The model under review builds one solid part; all positions refer to its coordinate system, in mm. A direction names the side the tool comes from. Round coordinates to 2 decimals unless told otherwise and drop trailing zeros. Order: outer loops, then holes, each group sorted by start corner. A loop starts at its lowest first (then second) coordinate and runs counter-clockwise, first axis right, second up. Notation, with made-up numbers: (-2.5, 26.25) -> (20.5, 26.25) arc R19 cw to (20.5, 34.25) -> close; hole circle Ø11 at (40.5, -10.75). An arc over 180 degrees is marked (long way). Use a Markdown table: item, result. Add a question column.
```python
from build123d import *

# Parameters (mm, degrees)
BOSS_EXTRUDE1_DEPTH = 2.975
SKETCH2_W           = 25.407464895
SKETCH2_H           = 9.803414335
BOSS_EXTRUDE2_DEPTH = 5.5
FILLET1_R           = 1
FILLET2_R           = 1
FILLET3_R           = 1
FILLET4_R           = 1
CUT_EXTRUDE3_DEPTH  = 10
SKETCH6_R           = 2.175
CUT_EXTRUDE4_DEPTH  = 10
SKETCH5_R           = 2.175
CUT_EXTRUDE2_DEPTH  = 10


with BuildPart() as part:
    # Sketch1 → Boss-Extrude1 (new body)
    with BuildSketch(Plane(origin=(0, 0, 0), x_dir=(1, 0, 0), z_dir=(0, 1, 0))):
        with BuildLine():
            Line((-23.171929825, 5.625877193), (2.228070175, 5.625877193))
            ThreePointArc((2.228070175, 5.625877193), (8.578070175, -0.724122807), (2.228070175, -7.074122807))
            Line((2.228070175, -7.074122807), (-23.171929825, -7.074122807))
            ThreePointArc((-23.171929825, -7.074122807), (-29.521929825, -0.724122807), (-23.171929825, 5.625877193))
        make_face()
    extrude(amount=BOSS_EXTRUDE1_DEPTH)

    # Sketch2 → Boss-Extrude2 (add)
    with BuildSketch(Plane.XY.offset(7.074122807)):
        with Locations((-10.460194126, 1.178603883)):
            Rectangle(SKETCH2_W, SKETCH2_H)
    extrude(amount=BOSS_EXTRUDE2_DEPTH)

    # Fillet1
    fillet1_edges = [part.edges().sort_by_distance(p)[0] for p in [
        (-23.163926573, 1.178603883, 12.574122807),
    ]]
    fillet(fillet1_edges, radius=FILLET1_R)

    # Fillet2
    fillet2_edges = [part.edges().sort_by_distance(p)[0] for p in [
        (2.243538322, 1.178603883, 12.574122807),
    ]]
    fillet(fillet2_edges, radius=FILLET2_R)

    # Fillet3
    fillet3_edges = [part.edges().sort_by_distance(p)[0] for p in [
        (-10.460194125, -3.723103285, 12.574122807),
        (-23.163926573, -3.723103285, 9.324122807),
        (-22.871033354, -3.723103285, 12.281229588),
        (2.243538322, -3.723103285, 9.324122807),
        (1.950645103, -3.723103285, 12.281229588),
    ]]
    fillet(fillet3_edges, radius=FILLET3_R)

    # Fillet4
    fillet4_edges = [part.edges().sort_by_distance(p)[0] for p in [
        (-23.163926573, 6.08031105, 9.324122807),
        (-22.871033354, 6.08031105, 12.281229588),
        (-10.460194125, 6.08031105, 12.574122807),
        (2.243538322, 6.08031105, 9.324122807),
        (1.950645103, 6.08031105, 12.281229588),
    ]]
    fillet(fillet4_edges, radius=FILLET4_R)

    # Sketch4 → Cut-Extrude3 (cut)
    with BuildSketch(Plane.XZ.offset(3.723103285)):
        Polygon((-15.163926573, 12.574122807), (-17.163926573, 12.574122807), (-16.163926519, 11.574122807), align=None)
        Polygon((-11.163926573, 12.574122807), (-13.163926573, 12.574122807), (-12.163926519, 11.574122807), align=None)
        Polygon((-7.163926573, 12.574122807), (-9.163926573, 12.574122807), (-8.163926519, 11.574122807), align=None)
        Polygon((-3.163926573, 12.574122807), (-5.163926573, 12.574122807), (-4.163926519, 11.574122807), align=None)
        Polygon((0.836073427, 12.574122807), (-1.163926573, 12.574122807), (-0.163926519, 11.574122807), align=None)
        Polygon((-21.163926573, 12.574122807), (-19.163926573, 12.574122807), (-20.163926519, 11.574122807), align=None)
    extrude(amount=-CUT_EXTRUDE3_DEPTH, mode=Mode.SUBTRACT)

    # Sketch6 → Cut-Extrude4 (cut)
    with BuildSketch(Plane(origin=(0, 2.975, 0), x_dir=(1, 0, 0), z_dir=(0, 1, 0))):
        with Locations(Location((-9.568561245, -0.724122807, 0), (0, 0, 270))):
            Circle(SKETCH6_R)
    extrude(amount=-CUT_EXTRUDE4_DEPTH, mode=Mode.SUBTRACT)

    # Sketch5 → Cut-Extrude2 (cut)
    with BuildSketch(Plane.XZ):
        with Locations((-9.989014044, 0.724122807)):
            Circle(SKETCH5_R)
    extrude(amount=-CUT_EXTRUDE2_DEPTH, mode=Mode.SUBTRACT)


solid = part.part
```
Q1. For faces 4 (the face through (-10, 0, -2)), 5 (the face through (2.244, 1, 9)), 6 (the face through (-3.67, 1.11, 12.07)), 7 (the face through (-6.14, -3.55, 12.14)), list the 3-axis set-ups (+Z, -Z, +X, -X, +Y, -Y) from which the entire face can be reached by the end or side of a thin tool; tool diameter is ignored.
Q2. Add section C-C, the plane y = -2.25. Give the boundary of the cut face in (x, z), then the cut area to 3 significant figures.
Q3. For pin 1 (4 mm diameter, centred on x = -13, z = -2, fed in from -Y); pin 2 (1.5 mm diameter, centred on x = -25.5, y = 5, fed in from -Z); pin 3 (1.5 mm diameter, centred on y = 4, z = 8.5, fed in from +X); pin 4 (10 mm diameter, centred on x = -18, z = -2, fed in from +Y) (3 decimals), all flat-tipped, find the tip position at first contact; note any pin that passes through.
Q4. Draft analysis for pull direction X (two halves, no side actions). For faces 1 (the face through (-14, 1, 12.574)), 2 (the face through (-12.67, 1.11, 12.08)), 3 (the face through (1.96, 5.78, 9.29)), state which applies: released by +X, released by -X, zero draft, split by the parting line, or undercut.
Q5. To check wall thickness, follow line 1 along Y through (x, z) = (-16, 4) (3 decimals); line 2 along X through (y, z) = (2.75, 8.5); line 3 along Z through (x, y) = (6, 0.5). State the ranges of each line that lie inside material, in increasing order.
Q6. Add section B-B, the plane z = 0.5. Give the boundary of the cut face in (x, y) (3 decimals).
Q7. Add section A-A, the plane z = 10.25. Give the boundary of the cut face in (x, y), then the cut area to 3 significant figures.
Return value:
| question | item | result |
|---|---|---|
| 1 | face 4 | -Z, +X, -X, -Y |
| 1 | face 5 | +Z, +X, +Y, -Y |
| 1 | face 6 | +Z, +Y, -Y |
| 1 | face 7 | +Z, +X, -X, -Y |
| 2 | outline | (-23.16, 7.07) -> (2.24, 7.07) -> (2.24, 11.57) arc R1 ccw to (1.24, 12.57) -> (0.84, 12.57) -> (-0.16, 11.57) -> (-1.16, 12.57) -> (-3.16, 12.57) -> (-4.16, 11.57) -> (-5.16, 12.57) -> (-7.16, 12.57) -> (-8.16, 11.57) -> (-9.16, 12.57) -> (-11.16, 12.57) -> (-12.16, 11.57) -> (-13.16, 12.57) -> (-15.16, 12.57) -> (-16.16, 11.57) -> (-17.16, 12.57) -> (-19.16, 12.57) -> (-20.16, 11.57) -> (-21.16, 12.57) -> (-22.16, 12.57) arc R1 ccw to (-23.16, 11.57) -> close |
| 2 | area | 133 mm² |
| 3 | pin 1 | y = 0 |
| 3 | pin 2 | through |
| 3 | pin 3 | x = 2.24 |
| 3 | pin 4 | y = 2.975 |
| 4 | face 1 | zero draft |
| 4 | face 2 | undercut |
| 4 | face 3 | released by +X |
| 5 | line 1 | 0 to 2.975 |
| 5 | line 2 | -23.16 to 2.24 |
| 5 | line 3 | -4.38 to 5.83 |
| 6 | outline | (-29.518, 0) -> (-12.152, 0) -> (-12.152, 2.975) -> (-29.518, 2.975) -> close; (-7.405, 0) -> (8.574, 0) -> (8.574, 2.975) -> (-7.405, 2.975) -> close |
| 7 | outline | (-23.16, -2.72) arc R1 ccw to (-22.16, -3.72) -> (1.24, -3.72) arc R1 ccw to (2.24, -2.72) -> (2.24, 5.08) arc R1 ccw to (1.24, 6.08) -> (-22.16, 6.08) arc R1 ccw to (-23.16, 5.08) -> close |
| 7 | area | 248 mm² |
